Verification items for this drawing (mm, ordinates from the low corner). Coordinates: 2 decimals unless noted, no trailing zeros. Order: outer loops, then holes, each group sorted by start corner. A loop starts at its lowest first (then second) coordinate and runs counter-clockwise, first axis right, second up. Notation, with made-up numbers: (13.5, 56) - (39.5, 56) arc R24 ccw to (39.5, 92) - close; hole circle Ø1 at (-22, 41.5). An arc over 180 degrees is marked (long way). One line per question, with ' | ' between items. Start each with the question number.
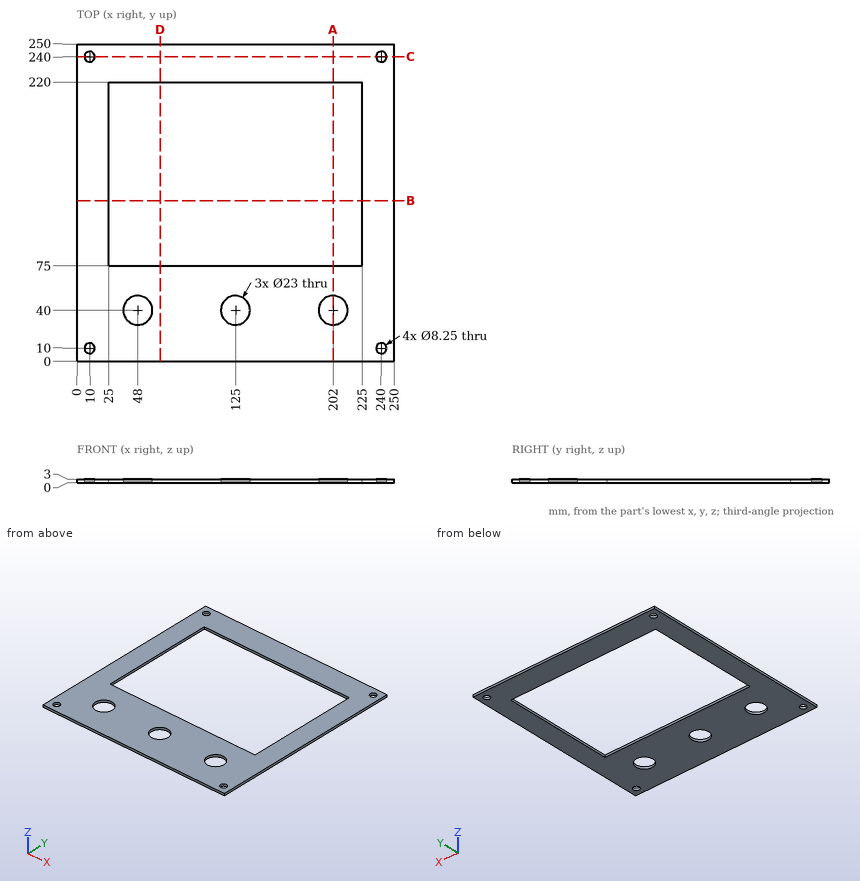
Item 1: Section check C-C (y = 240). Record the cut outline in (x, z) (3 decimals).
Item 2: Section check B-B (y = 126.5). Record the cut outline in (x, z).
Item 3: Thickness scan on probe 1 along Y at (x, z) = (48, 1.7); probe 2 along X at (y, z) = (39.5, 2); probe 3 along X at (y, z) = (34.5, 1.45). Record the ranges inside material, lowest first. Write a range as from..to.
Item 4: Section check A-A (x = 202). Record the cut outline in (y, z), then the cut area to 3 significant figures.
Item 5: Section check D-D (x = 65.5). Record the cut outline in (y, z), then the cut area to 3 significant figures.
Completed:
1) outline: (0, 0) - (5.875, 0) - (5.875, 3) - (0, 3) - close; (14.125, 0) - (235.875, 0) - (235.875, 3) - (14.125, 3) - close; (244.125, 0) - (250, 0) - (250, 3) - (244.125, 3) - close
2) outline: (0, 0) - (25, 0) - (25, 3) - (0, 3) - close; (225, 0) - (250, 0) - (250, 3) - (225, 3) - close
3) probe 1: y = 0..28.5, 51.5..75, 220..250 | probe 2: x = 0..36.51, 59.49..113.51, 136.49..190.51, 213.49..250 | probe 3: x = 0..37.9, 58.1..114.9, 135.1..191.9, 212.1..250
4) outline: (0, 0) - (28.5, 0) - (28.5, 3) - (0, 3) - close; (51.5, 0) - (75, 0) - (75, 3) - (51.5, 3) - close; (220, 0) - (250, 0) - (250, 3) - (220, 3) - close | area: 246 mm^2
5) outline: (0, 0) - (75, 0) - (75, 3) - (0, 3) - close; (220, 0) - (250, 0) - (250, 3) - (220, 3) - close | area: 315 mm^2
